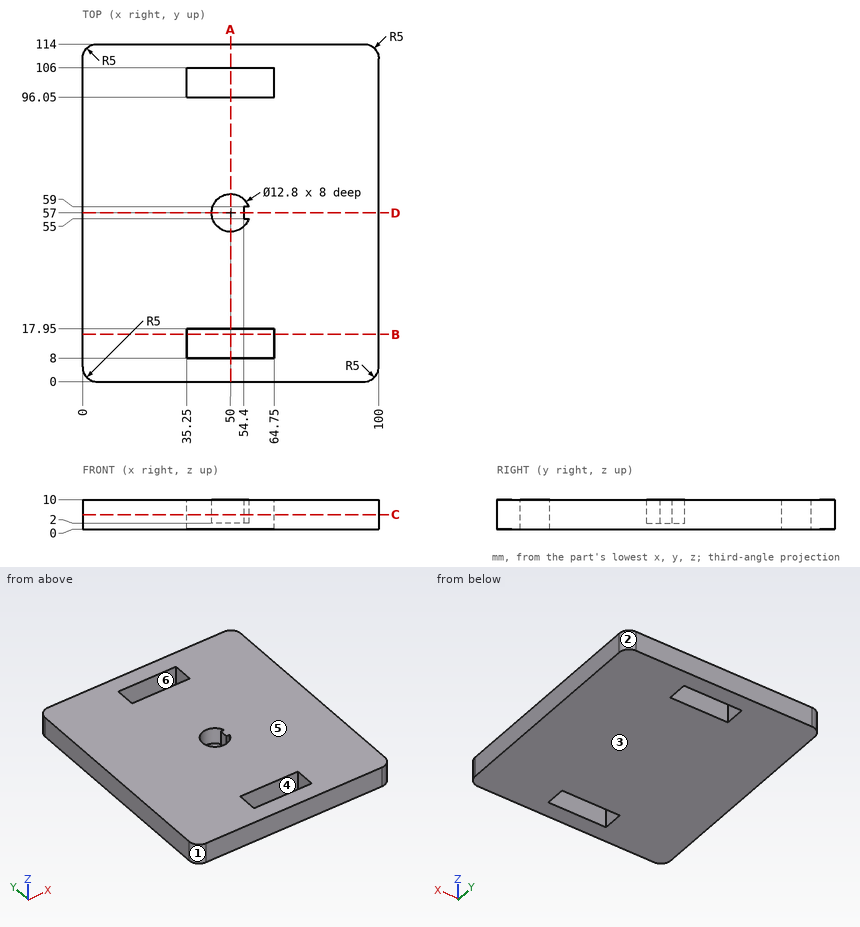
Geometry: see drawing. Coordinates: mm, zero at the bounding-box minimum. A direction names the side the tool comes from. Coordinates: 2 decimals unless noted, no trailing zeros. Loops run counter-clockwise (first coordinate to the right, second up) from the corner with the lowest first, then second, coordinate; pieces in that order, holes last. Notation, with made-up numbers: M 34,53 L 75,53 A25 cw 75,84 Z; hole C -26.75,12.25 d7. An arc over 180 degrees is marked long. Answer in a Markdown table with one row per item.
1. Draft query along X for the marked faces 1, 2, 3 and 4. Return one class per face: pulls with the +X half, pulls with the -X half, needs draft (parallel to the pull), parting line crosses it, or undercut.
Response:
| item | result |
|---|---|
| face 1 | pulls with the -X half |
| face 2 | pulls with the +X half |
| face 3 | needs draft |
| face 4 | undercut |
2. Section C-C, the plane z = 5. Output: boundary loops of the cut face in (x, y), then the cut area to 3 significant figures.
Response:
| item | result |
|---|---|
| outline | M 0,5 A5 ccw 5,0 L 95,0 A5 ccw 100,5 L 100,109 A5 ccw 95,114 L 5,114 A5 ccw 0,109 Z; hole M 35.25,8 L 64.75,8 L 64.75,17.95 L 35.25,17.95 Z; hole M 35.25,96.05 L 64.75,96.05 L 64.75,106 L 35.25,106 Z; hole M 54.4,55 L 54.4,59 L 56.08,59 A6.4 ccw long 56.08,55 Z |
| area | 10,700 mm2 |
3. Section B-B, the plane y = 16. Output: boundary loops of the cut face in (x, z), then the cut area to 3 significant figures.
Response:
| item | result |
|---|---|
| outline | M 0,0 L 35.25,0 L 35.25,10 L 0,10 Z; M 64.75,0 L 100,0 L 100,10 L 64.75,10 Z |
| area | 705 mm2 |
4. Material intervals for line 1 (Y direction, x = 50, z = 7.25); line 2 (Y direction, x = 42, z = 3); line 3 (X direction, y = 57, z = 7.75), sorted ascending.
Response:
| item | result |
|---|---|
| line 1 | y = 0 to 8, 17.95 to 50.6, 63.4 to 96.05, 106 to 114 |
| line 2 | y = 0 to 8, 17.95 to 96.05, 106 to 114 |
| line 3 | x = 0 to 43.6, 54.4 to 100 |
5. Reachability of the marked faces 5 and 6 from +Z, -Z, +X, -X, +Y, -Y: full face, straight path, thin tool, end or side. Return the list, or none.
Response:
| item | result |
|---|---|
| face 5 | +Z, +X, -X, +Y, -Y |
| face 6 | +Z, -Z |
6. Section D-D, the plane y = 57. Output: boundary loops of the cut face in (x, z), then the cut area to 3 significant figures.
Response:
| item | result |
|---|---|
| outline | M 0,0 L 100,0 L 100,10 L 54.4,10 L 54.4,2 L 43.6,2 L 43.6,10 L 0,10 Z |
| area | 914 mm2 |
7. Section A-A, the plane x = 50. Output: boundary loops of the cut face in (y, z), then the cut area to 3 significant figures.
Response:
| item | result |
|---|---|
| outline | M 0,0 L 8,0 L 8,10 L 0,10 Z; M 17.95,0 L 96.05,0 L 96.05,10 L 63.4,10 L 63.4,2 L 50.6,2 L 50.6,10 L 17.95,10 Z; M 106,0 L 114,0 L 114,10 L 106,10 Z |
| area | 839 mm2 |
